Here's the drawing with two shaded views (mm, measured from the low corner). I have some questions. A direction names the side the tool comes from. Give positions to 0.01 mm unless a question says otherwise; leave off trailing zeros. Loops run counter-clockwise (first coordinate to the right, second up) from the corner with the lowest first, then second, coordinate; pieces in that order, holes last.
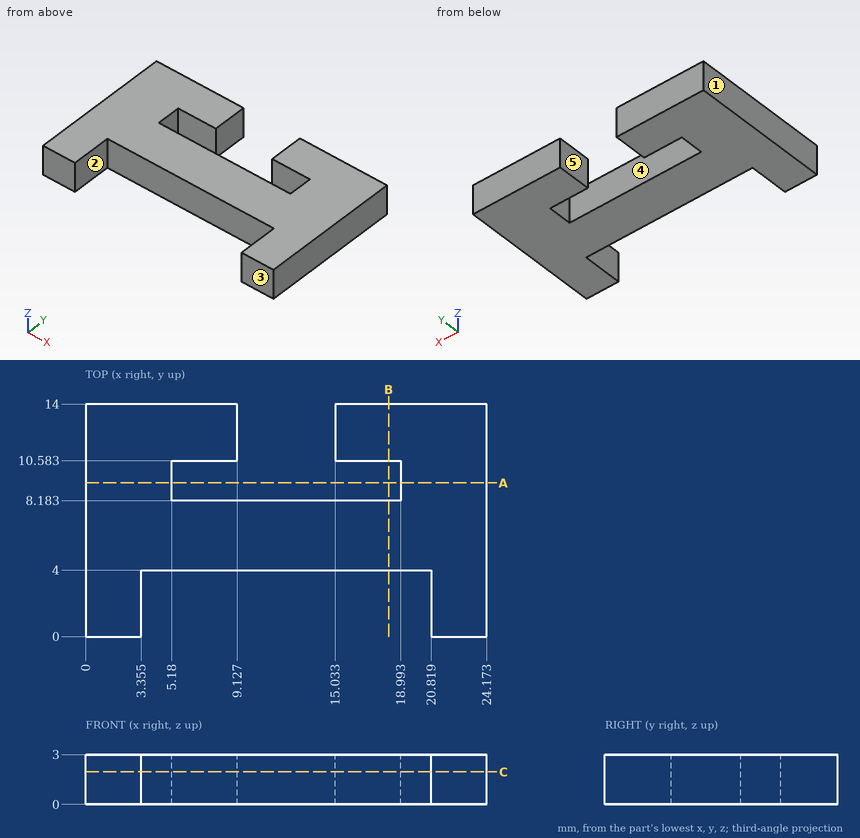
(1) Suppose I cut it at A-A on y = 9.25. List the corners of the cut face in (x, z) for me, plus the area to 3 significant figures.
Returned:
outline: (0, 0) - (5.18, 0) - (5.18, 3) - (0, 3) - close; (18.99, 0) - (24.17, 0) - (24.17, 3) - (18.99, 3) - close
area: 31.1 mm2
(2) Suppose I cut it at B-B on x = 18.25. List the corners of the cut face in (y, z) for me, plus the area to 3 significant figures.
Returned:
outline: (4, 0) - (8.18, 0) - (8.18, 3) - (4, 3) - close; (10.58, 0) - (14, 0) - (14, 3) - (10.58, 3) - close
area: 22.8 mm2
(3) Please list where these lines run through material, in increasing order: probe 1 along Y at (x, z) = (8, 1.2); probe 2 along X at (y, z) = (9.25, 1.75); probe 3 along X at (y, z) = (12.25, 1).
Returned:
probe 1: y = 4 to 8.18, 10.58 to 14
probe 2: x = 0 to 5.18, 18.99 to 24.17
probe 3: x = 0 to 9.13, 15.03 to 24.17
(4) Will this pin go through, and if not, where does the flat tip stop? P1, Ø1.5, axis at x = 10, z = 1, coming from the -Y side.
Returned:
P1: stops at y = 4
(5) Suppose I cut it at C-C on z = 1.95. List the corners of the cut face in (x, y) for me (1 decimal).
Returned:
outline: (0, 0) - (3.4, 0) - (3.4, 4) - (20.8, 4) - (20.8, 0) - (24.2, 0) - (24.2, 14) - (15, 14) - (15, 10.6) - (19, 10.6) - (19, 8.2) - (5.2, 8.2) - (5.2, 10.6) - (9.1, 10.6) - (9.1, 14) - (0, 14) - close
(6) Which directions (+Z, -Z, +X, -X, +Y, -Y) give clear straight access to the entire face, cutting with the end or side of a thin tool? Please do the marked faces 1, 2, 3, 4 and 5.
Returned:
face 1: +Z, -Z, -X, +Y, -Y
face 2: +Z, -Z, -Y
face 3: +Z, -Z, +X, -X, -Y
face 4: +Z, -Z
face 5: +Z, -Z, +Y
